from build123d import *

# Parameters (mm, degrees)
SKETCH_1_R         = 2.5
EXTRUDE_2_DEPTH    = 170
SCALE1_SCALE       = 2.5
SKETCH1_W          = 66.249560654
SKETCH1_H          = 85.957176857
CUT_EXTRUDE1_DEPTH = 50


with BuildPart() as part:
    # 草图1 → 凸台-拉伸2 (new body)
    with BuildSketch(Plane.XY):
        with BuildLine():
            Line((5.5, -8.2), (5.5, -6.560660172))
            Line((5.5, -6.560660172), (2.939339828, -4))
            Line((2.939339828, -4), (-2.939339828, -4))
            Line((-2.939339828, -4), (-5.5, -6.560660172))
            Line((-5.5, -6.560660172), (-5.5, -8.2))
            Line((-5.5, -8.2), (-3.1, -8.2))
            Line((-3.1, -8.2), (-3.1, -10))
            Line((-3.1, -10), (-8.5, -10))
            ThreePointArc((-8.5, -10), (-9.560660172, -9.560660172), (-10, -8.5))
            Line((-10, -8.5), (-10, -3.1))
            Line((-10, -3.1), (-8.2, -3.1))
            Line((-8.2, -3.1), (-8.2, -5.5))
            Line((-8.2, -5.5), (-6.560660172, -5.5))
            Line((-6.560660172, -5.5), (-4, -2.939339828))
            Line((-4, -2.939339828), (-4, 2.939339828))
            Line((-4, 2.939339828), (-6.560660172, 5.5))
            Line((-6.560660172, 5.5), (-8.2, 5.5))
            Line((-8.2, 5.5), (-8.2, 3.1))
            Line((-8.2, 3.1), (-10, 3.1))
            Line((-10, 3.1), (-10, 8.5))
            ThreePointArc((-10, 8.5), (-9.560660172, 9.560660172), (-8.5, 10))
            Line((-8.5, 10), (-3.1, 10))
            Line((-3.1, 10), (-3.1, 8.2))
            Line((-3.1, 8.2), (-5.5, 8.2))
            Line((-5.5, 8.2), (-5.5, 6.560660172))
            Line((-5.5, 6.560660172), (-2.939339828, 4))
            Line((-2.939339828, 4), (2.939339828, 4))
            Line((2.939339828, 4), (5.5, 6.560660172))
            Line((5.5, 6.560660172), (5.5, 8.2))
            Line((5.5, 8.2), (3.1, 8.2))
            Line((3.1, 8.2), (3.1, 10))
            Line((3.1, 10), (8.5, 10))
            ThreePointArc((8.5, 10), (9.560660172, 9.560660172), (10, 8.5))
            Line((10, 8.5), (10, 3.1))
            Line((10, 3.1), (8.2, 3.1))
            Line((8.2, 3.1), (8.2, 5.5))
            Line((8.2, 5.5), (6.560660172, 5.5))
            Line((6.560660172, 5.5), (4, 2.939339828))
            Line((4, 2.939339828), (4, -2.939339828))
            Line((4, -2.939339828), (6.560660172, -5.5))
            Line((6.560660172, -5.5), (8.2, -5.5))
            Line((8.2, -5.5), (8.2, -3.1))
            Line((8.2, -3.1), (10, -3.1))
            Line((10, -3.1), (10, -8.5))
            ThreePointArc((10, -8.5), (9.560660172, -9.560660172), (8.5, -10))
            Line((8.5, -10), (3.1, -10))
            Line((3.1, -10), (3.1, -8.2))
            Line((3.1, -8.2), (5.5, -8.2))
        make_face()
        Circle(SKETCH_1_R, mode=Mode.SUBTRACT)
    extrude(amount=-EXTRUDE_2_DEPTH)


with BuildPart() as part_1:
    # Scale1: scaled about (0, 0, 0)
    add(part.part.scale(SCALE1_SCALE))

    # Sketch1 → Cut-Extrude1 (cut)
    with BuildSketch(Plane(origin=(0, 200, -200), x_dir=(1, 0, 0), z_dir=(1.0176525195173148e-14, 0.7071067811865488, -0.7071067811865464))):
        with Locations((1.305108883, 276.28516192)):
            Rectangle(SKETCH1_W, SKETCH1_H)
    cut_extrude1 = extrude(amount=CUT_EXTRUDE1_DEPTH, mode=Mode.SUBTRACT)

    # Mirror1: Cut-Extrude1 across plane
    add(cut_extrude1.mirror(Plane.XY.offset(-212.5)), mode=Mode.SUBTRACT)


solid = part_1.part
Can you work these out from the model? Positions are in its coordinate system, mm. A direction names the side the tool comes from. Coordinates: 2 decimals unless noted, no trailing zeros. Write each loop counter-clockwise with the first axis right and the second up, starting at its lowest first coordinate (ties: lowest second). Pieces come first, ordered by that corner, then holes. Notation, with made-up numbers: (-2, 26) -> (46, 26) arc R14 ccw to (46, 46) -> close; hole circle Ø3 at (-3, 1). An arc over 180 degrees is marked (long way). Answer as CSV lines item,"result".
1) If we mould it in two halves opening along X, with no side actions, what happens to faces 1 (the cylindrical face through (5.96, 1.88, -209.71)), 2 (the flat face through (15, -25, -210)), 3 (the flat face through (25, 15, -210))? For each: +X half, -X half, draft (parallel to the pull), parting line (faces both ways), or undercut.
Check result:
face 1,"undercut"
face 2,"draft"
face 3,"+X half"
2) If we section it at A-A on x = 0: Please give me the cut outline in (y, z), then the cut area to 3 significant figures.
Check result:
outline,"(-10, -410) -> (-6.25, -406.25) -> (-6.25, -18.75) -> (-10, -15) -> close; (6.25, -393.75) -> (10, -390) -> (10, -35) -> (6.25, -31.25) -> close"
area,"2,810 mm²"
3) On a 3-axis mill with a long thin cutter (end or side, diameter ignored), from which of +Z, -Z, +X, -X, +Y, -Y can I reach the whole of each face in a straight line? I mean faces 4 (the flat face through (0, -10, -210)), 5 (the flat face through (10, 0, -210)), 6 (the flat face through (-10, 0, -210)), 7 (the flat face through (0, 10, -210)). Say none if no direction works.
Check result:
face 4,"+Z, -Z, -Y"
face 5,"+Z, -Z, +X"
face 6,"+Z, -Z, -X"
face 7,"+Z, -Z, +Y"
4) Will these pins go through, and if not, where does the flat tip stop? P1, Ø16, axis at x = 0, y = 0, coming from the -Z side; P2, Ø3.5, axis at x = 23, z = -139.5, coming from the -Y side; P3, Ø1.4, axis at y = -22.5, z = -108.5, coming from the +X side; P4, Ø1, axis at x = -15.5, y = -17, coming from the -Z side.
Check result:
P1,"z = -408"
P2,"y = -25"
P3,"x = 24.96"
P4,"z = -417.5"
5) If we section it at B-B on y = 0: Please give me the cut outline in (x, z).
Check result:
outline,"(-10, -400) -> (-6.25, -400) -> (-6.25, -25) -> (-10, -25) -> close; (6.25, -400) -> (10, -400) -> (10, -25) -> (6.25, -25) -> close"
6) If I drill on line 1 (Y direction, x = -17, z = -334); line 2 (X direction, y = 0, z = -114), over which ranges is the centre line in solid material (lowest first)? Write a range as from..to.
Check result:
line 1,"-25..-13.75, 13.75..25"
line 2,"-10..-6.25, 6.25..10"
